Verification items for the finished model (mm, model axes). A direction names the side the tool comes from. Round coordinates to 2 decimals unless told otherwise and drop trailing zeros. Loops run counter-clockwise (first coordinate to the right, second up) from the corner with the lowest first, then second, coordinate; pieces in that order, holes last.
from build123d import *

# Parameters (mm, degrees)
SKETCH3_R = 1
SKETCH4_R = 1
SKETCH6_R = 1


with BuildPart() as part:
    # Sweep1: sweep along a path in Sketch1
    with BuildLine(Plane.XY) as sweep1_path:
        Line((0, 0), (0, -10.694484018))
        ThreePointArc((0, -10.694484018), (-2.928932188, -17.76555183), (-10, -20.694484018))
        Line((-10, -20.694484018), (-12.508437971, -20.694484018))
    # Sketch3 → Sweep1 (sweep)
    with BuildSketch(Plane(origin=(0, 0, 0), x_dir=(1, 0, 0), z_dir=(0, 1, 0))):
        Circle(SKETCH3_R)
    sweep(path=sweep1_path.line)

    # Sweep2: sweep along a path in Sketch2
    with BuildLine(Plane(origin=(0, -20.694484018, 0), x_dir=(1, 0, 0), z_dir=(0, 1, 0))) as sweep2_path:
        Line((-12.508437971, 0), (-13.348220683, 0))
        ThreePointArc((-13.348220683, 0), (-15.469541026, 0.878679656), (-16.348220683, 3))
        Line((-16.348220683, 3), (-16.348220683, 39.916632526))
    # Sketch4 → Sweep2 (sweep)
    with BuildSketch(Plane.ZY.offset(12.508437971)):
        with Locations((0, -20.694484018)):
            Circle(SKETCH4_R)
    sweep(path=sweep2_path.line)

    # Sweep3: sweep along a path in Sketch5
    with BuildLine(Plane(origin=(-16.348220683, 0, 0), x_dir=(0, 0, -1), z_dir=(1, 0, 0))) as sweep3_path:
        Line((39.916632526, -20.694484018), (42.629508897, -20.694484018))
        ThreePointArc((42.629508897, -20.694484018), (44.750829241, -21.573163675), (45.629508897, -23.694484018))
        Line((45.629508897, -23.694484018), (45.629508897, -26.831314156))
    # Sketch6 → Sweep3 (sweep)
    with BuildSketch(Plane(origin=(0, 0, -39.916632526), x_dir=(-1, 0, 0), z_dir=(0, 0, -1))):
        with Locations((16.348220683, -20.694484018)):
            Circle(SKETCH6_R)
    sweep(path=sweep3_path.line)


solid = part.part
1. Section check A-A (y = -5.5). Enter the section's corners in (x, z).
2. Scan lines: L1, parallel to X at y = -21, z = -4.5; L2, parallel to Z at x = -1, y = -12.5. Record each from-to range of solid material in increasing order.
3. Section check B-B (z = -5). Enter the section's corners in (x, y).
4. Tool access check on faces 4 (the face through (-16, -26.831, -46)), 5 (the face through (-16.131, -25.285, -44.653)), 6 (the face through (0, -5, -1)). Record the directions out of +Z, -Z, +X, -X, +Y, -Y that give a thin tool (end or side, any length) a straight path to the whole face; none if there is none.
5. Release check for a two-part mould opening along Z. For faces 1 (the face through (-11.698, -21.623, 0.372)), 2 (the face through (-16.218, -19.703, -23.092)), 3 (the face through (0, 0, 0)) record: released by +Z, released by -Z, zero draft, split by the parting line, or undercut.
6. Gauge pin test, flat ends, axial feed: P1, Ø1, axis at x = -8, y = -18.5, coming from the -Z side; P2, Ø3, axis at x = -2, y = -5, coming from the -Z side; P3, Ø10, axis at x = -6.5, y = -19, coming from the +Z side. Record the tip position at first contact, or that the pin passes through.
Taken from the geometry:
1. outline: circle Ø2 at (0, 0)
2. L1: x = -17.3 to -15.4
2. L2: z = -0.57 to 0.57
3. outline: circle Ø2 at (-16.35, -20.69)
4. face 4: +Z, -Z, +X, -X, -Y
4. face 5: -Y
4. face 6: +Y
5. face 1: split by the parting line
5. face 2: undercut
5. face 3: zero draft
6. P1: passes through
6. P2: stops at z = -0.87
6. P3: stops at z = 1
